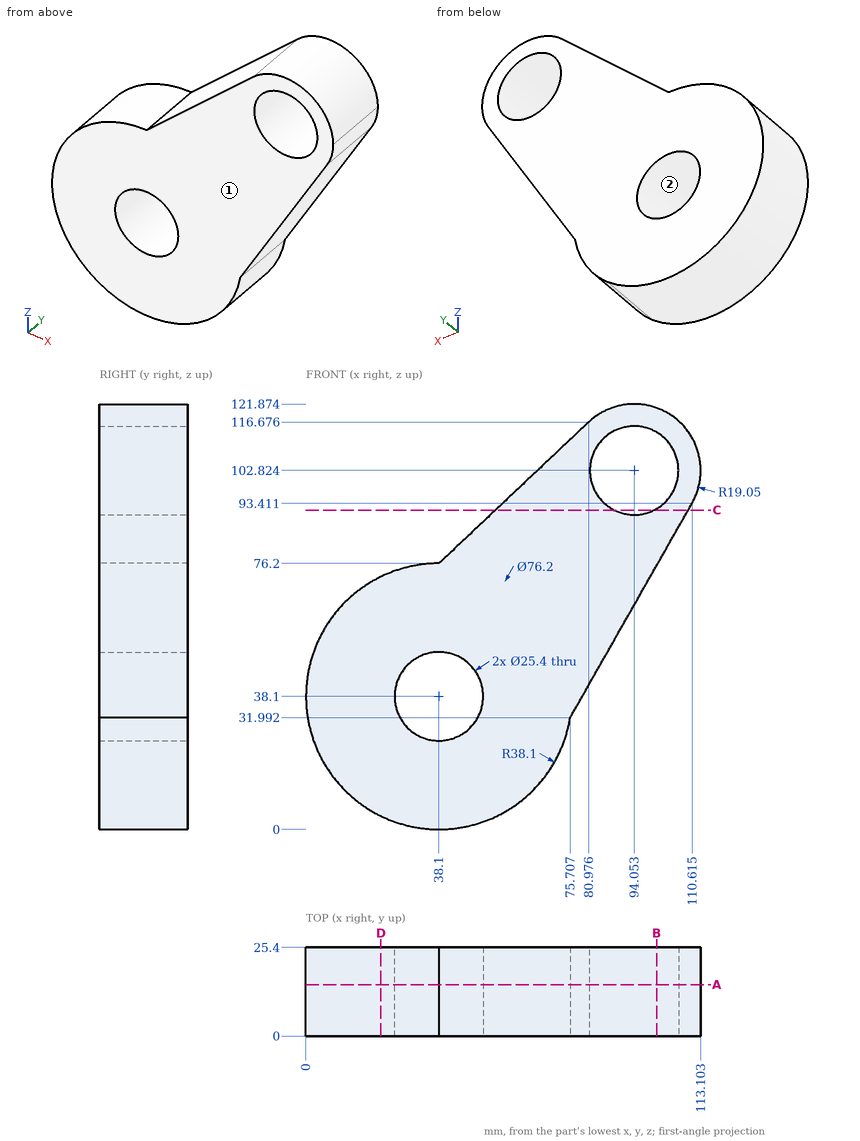
Answer from the drawing. Dimensions are ordinates in mm from the lowest x, y and z of the part. Coordinates: 2 decimals unless noted, no trailing zeros. Write each loop counter-clockwise with the first axis right and the second up, starting at its lowest first coordinate (ties: lowest second). Pieces come first, ordered by that corner, then holes. Notation, with made-up numbers: (51, 23.5) - (86, 23.5) arc R24 cw to (86, 58.5) - close; hole circle Ø5 at (-11, -4.5). An arc over 180 degrees is marked (long way). Return JSON: item names as keys, results as strings.
1. The part is cut by section C-C on z = 91.5. Determine the outline of the cut face in (x, y).
Final values:
{"outline": "(54.31, 0) - (88.3, 0) - (88.3, 25.4) - (54.31, 25.4) - close; (99.8, 0) - (109.53, 0) - (109.53, 25.4) - (99.8, 25.4) - close"}
2. Consider line 1 along Z through (x, y) = (47.5, 5.25) (1 decimal); line 2 along X through (y, z) = (9.75, 105) (1 decimal); line 3 along X through (y, z) = (13, 37.5) (1 decimal). Determine where each line is inside the solid, lowest interval first.
Final values:
{"line 1": "1.2 to 29.6, 46.6 to 85.1", "line 2": "68.6 to 81.5, 106.6 to 113", "line 3": "0 to 25.4, 50.8 to 78.8"}
3. The part is cut by section B-B on x = 100.5. Determine the outline of the cut face in (y, z).
Final values:
{"outline": "(0, 75.61) - (25.4, 75.61) - (25.4, 91.88) - (0, 91.88) - close; (0, 113.77) - (25.4, 113.77) - (25.4, 120.75) - (0, 120.75) - close"}
4. Each of these flat-tipped pins is pushed along its axis until it touches: pin 1 Ø12 at (y, z) = (18, 45.5) entering from -X; pin 2 Ø1 at (x, y) = (99.5, 11) entering from -Z (1 decimal); pin 3 Ø8 at (x, y) = (56, 21.5) entering from +Z (1 decimal). Where does it stop, or does it pass through?
Final values:
{"pin 1": "x = 0.03", "pin 2": "z = 73", "pin 3": "z = 96.9"}
5. The part is cut by section D-D on x = 21.5. Determine the outline of the cut face in (y, z), then the cut area to 3 significant figures.
Final values:
{"outline": "(0, 3.81) - (25.4, 3.81) - (25.4, 72.39) - (0, 72.39) - close", "area": "1,740 mm^2"}
6. For a pull along Z with two mould halves and no side action, classify the marked faces 1 and 2 as +Z half, -Z half, draft (parallel to the pull), parting line (faces both ways), or undercut.
Final values:
{"face 1": "draft", "face 2": "undercut"}
7. The part is cut by section A-A on y = 14.75. Count the separate pieces of the cut face and the enclosed holes in it, then the cut area to 3 significant figures.
Final values:
{"separate pieces": "1", "enclosed holes": "2", "area": "6,490 mm^2"}
